```python
from build123d import *

# Parameters (mm, degrees)
F1_W     = 127
F1_H     = 127
F2_DEPTH = 63.5
F3_R     = 38.1
F4_DEPTH = 50.8
F5_R     = 38.1
F6_DEPTH = 38.1


# Not quite as in the source:
# - a variable given as a bare number and used for a length is read in inches; the dataset says mm whatever the document's units were


with BuildPart() as f2:
    # F1 (on Top) → F2 (new body, symmetric)
    with BuildSketch(Plane.XY):
        Rectangle(F1_W, F1_H)
    extrude(amount=F2_DEPTH, both=True)

    # F3 (on face) → F4 (cut)
    with BuildSketch(Plane.XZ.offset(63.5)):
        Circle(F3_R)
    extrude(amount=-F4_DEPTH, mode=Mode.SUBTRACT)

    # F5 (on face) → F6 (join)
    with BuildSketch(Plane(origin=(0, 63.5, 0), x_dir=(-1, 0, 0), z_dir=(0, 1, 0))):
        Circle(F5_R)
    extrude(amount=F6_DEPTH)


solid = f2.part
```
Model file for the job. Use its own axes, mm. A direction names the side the tool comes from. Coordinates: 2 decimals unless noted, no trailing zeros. Write each loop counter-clockwise with the first axis right and the second up, starting at its lowest first coordinate (ties: lowest second). Pieces come first, ordered by that corner, then holes. Notation, with made-up numbers: (23, 48.5) - (41, 48.5) arc R10 ccw to (41, 60.5) - close; hole circle Ø2 at (19, 7.5). An arc over 180 degrees is marked (long way). One line per question, with ' | ' between items. Start each with the question number.
Q1. Pull direction X, two halves, no side cores. Call faces 1 (the face through (1, 101.6, 1)), 2 (the face through (-30.235, -38.456, -23.183)), 3 (the face through (-1, -12.7, 1)), 4 (the face through (-63.5, -1, 1)): pulls with the +X half, pulls with the -X half, needs draft (parallel to the pull), parting line crosses it, or undercut.
Q2. Cut at D-D, the plane z = -42.5. List the corners of the cut face in (x, y), then the cut area to 3 significant figures.
Q3. Cut at A-A, the plane x = 0. List the corners of the cut face in (y, z), then the cut area to 3 significant figures.
Q4. Cut at B-B, the plane z = 0. List the corners of the cut face in (x, y).
Q5. Cut at C-C, the plane y = 67. List the corners of the cut face in (x, z).
Q6. 3-axis set-ups, long thin cutter, end or side, ignore diameter. For faces 5 (the face through (27, -63.5, 29)), 6 (the face through (27, 63.5, 29)): which of +Z, -Z, +X, -X, +Y, -Y reach the whole face in a straight line?
Q7. Pin check, flat tips, straight feed: pin 1 (10 mm diameter, centred on x = -45.5, z = -3.5, fed in from +Y); pin 2 (2 mm diameter, centred on x = 3.5, z = -31, fed in from -Y); pin 3 (12 mm diameter, centred on x = -22.5, y = 70, fed in from +Z). Stop position of each tip, or through.
Q8. Drill centre lines: line 1 (Z direction, x = 0, y = -42); line 2 (Y direction, x = 1.5, z = -26); line 3 (Y direction, x = -25.5, z = -32.5). Where is each one in solid material? Low to high. Write a range as [from, to].
Answer below:
1) face 1: needs draft | face 2: undercut | face 3: undercut | face 4: pulls with the -X half
2) outline: (-63.5, -63.5) - (63.5, -63.5) - (63.5, 63.5) - (-63.5, 63.5) - close | area: 16,100 mm^2
3) outline: (-63.5, -63.5) - (63.5, -63.5) - (63.5, -38.1) - (101.6, -38.1) - (101.6, 38.1) - (63.5, 38.1) - (63.5, 63.5) - (-63.5, 63.5) - (-63.5, 38.1) - (-12.7, 38.1) - (-12.7, -38.1) - (-63.5, -38.1) - close | area: 15,200 mm^2
4) outline: (-63.5, -63.5) - (-38.1, -63.5) - (-38.1, -12.7) - (38.1, -12.7) - (38.1, -63.5) - (63.5, -63.5) - (63.5, 63.5) - (38.1, 63.5) - (38.1, 101.6) - (-38.1, 101.6) - (-38.1, 63.5) - (-63.5, 63.5) - close
5) outline: circle Ø76.2 at (0, 0)
6) face 5: +Z, -Z, +X, -X, -Y | face 6: +Y
7) pin 1: y = 63.5 | pin 2: y = -12.7 | pin 3: z = 34.34
8) line 1: [-63.5, -38.1], [38.1, 63.5] | line 2: [-12.7, 101.6] | line 3: [-63.5, 63.5]
